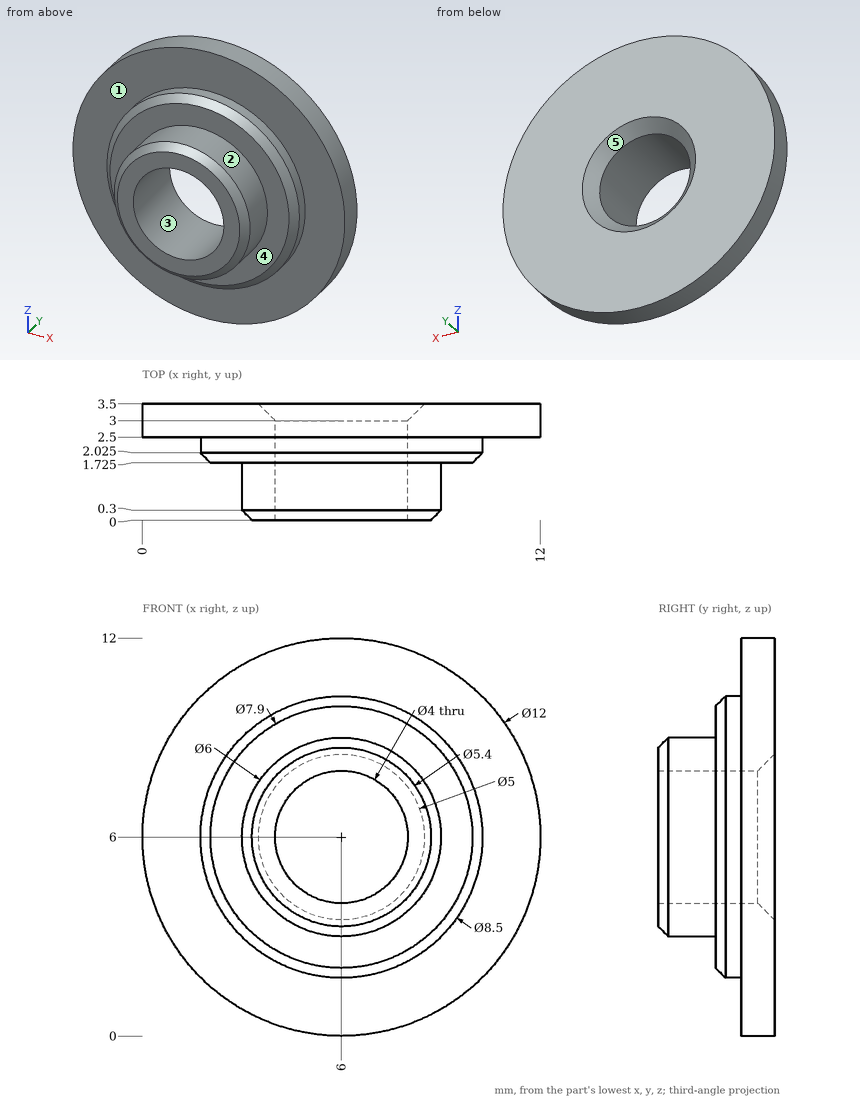
Answer from the drawing. Dimensions are ordinates in mm from the lowest x, y and z of the part. A direction names the side the tool comes from. Give positions to 0.01 mm unless a question says otherwise; leave off trailing zeros.
(1) Straight lines are drawn through the part: L1, parallel to X at y = 1, z = 6; L2, parallel to Y at x = 10, z = 2.5. For each, find the intervals that lie inside material, in ascending order.
(2) For the marked faces 4 and 5, determine the directions among +Z, -Z, +X, -X, +Y, -Y from which every point of the face is accessible in a straight line to the end or side of a thin tool.
(3) For a pull along Z with two mould halves and no side action, classify the marked faces 1, 2 and 3 as released by +Z, released by -Z, zero draft, split by the parting line, or undercut.
(4) Given pin 1 (1 mm diameter, centred on x = 2, z = 5, fed in from -Y) (1 decimal), flat-ended and moving along its own axis, determine where the tip first touches the part or whether it passes through.
Result sheet:
1. L1: x = 3 to 4, 8 to 9
1. L2: y = 2.5 to 3.5
2. face 4: -Y
2. face 5: +Y
3. face 1: zero draft
3. face 2: split by the parting line
3. face 3: undercut
4. pin 1: stops at y = 1.7
